The model under review builds one solid part; all positions refer to its coordinate system, in mm. Face numbers are marked on the shaded views. Give positions to 0.01 mm unless a question says otherwise; leave off trailing zeros. Order: outer loops, then holes, each group sorted by start corner. A loop starts at its lowest first (then second) coordinate and runs counter-clockwise, first axis right, second up. Notation, with made-up numbers: M 43.5,78.5 L 62.5,78.5 A25 ccw 62.5,102.5 Z; hole C 19.25,63 d4. An arc over 180 degrees is marked long. One line per question, with ' | ' between items. Start each with the question number.
1. Wall thickness on L1, parallel to Y at x = 0, z = 8.8; L2, parallel to X at y = -21.5, z = 8.5; L3, parallel to X at y = 38.5, z = 6.5: over which ranges is each line inside the solid? List them lowest first.
2. The part is to be moulded in two halves that separate along Y. For the marked faces 1, 2 and 3, say which applies: +Y half, -Y half, draft (parallel to the pull), parting line (faces both ways), or undercut.
3. Insertion check: P1, Ø6, axis at y = 19.5, z = 9, coming from the +X side; P2, Ø4, axis at x = -66.57, y = 21.63, coming from the -Z side; P3, Ø3, axis at x = -19.5, z = 7, coming from the +Y side; P4, Ø6, axis at y = 38, z = 2.5, coming from the -X side. Each pin has a flat end and moves straight along its axis. Give the tip position at first contact, or say it passes through.
4. We need section D-D on z = 3.75. Write out the cut boundary in (x, y), then the cut area to 3 significant figures.
5. We need section B-B on y = 33. Write out the cut boundary in (x, z), then the cut area to 3 significant figures.
6. We need section C-C on x = -53. Write out the cut boundary in (y, z).
7. We need section A-A on x = 0. Write out the cut boundary in (y, z), then the cut area to 3 significant figures.
```python
from build123d import *

# Parameters (mm, degrees)
SKETCH2_R           = 75
BOSS_EXTRUDE1_DEPTH = 10
SKETCH3_R           = 55
CUT_EXTRUDE1_DEPTH  = 10
SKETCH6_R           = 3
CUT_EXTRUDE2_DEPTH  = 3
SKETCH5_R           = 2.5
CUT_EXTRUDE3_DEPTH  = 107.536378763
CIRPATTERN2_COUNT   = 5


with BuildPart() as part:
    # Sketch2 → Boss-Extrude1 (new body)
    with BuildSketch(Plane(origin=(0, 0, 0), x_dir=(0, 1, 0), z_dir=(0, 0, 1))):
        with Locations(Location((0, 0, 0), (0, 0, 270))):
            Circle(SKETCH2_R)
    extrude(amount=BOSS_EXTRUDE1_DEPTH)

    # Sketch3 → Cut-Extrude1 (cut)
    with BuildSketch(Plane.XY.offset(10)):
        Circle(SKETCH3_R)
    extrude(amount=-CUT_EXTRUDE1_DEPTH, mode=Mode.SUBTRACT)

    # Sketch6 → Cut-Extrude2 (cut)
    with BuildSketch(Plane.XY.offset(10)):
        with Locations((0, 70)):
            Circle(SKETCH6_R)
    cut_extrude2 = extrude(amount=-CUT_EXTRUDE2_DEPTH, mode=Mode.SUBTRACT)

    # Sketch5 → Cut-Extrude3 (cut, through all)
    with BuildSketch(Plane.XY.offset(10)):
        with Locations((0, 70)):
            Circle(SKETCH5_R)
    cut_extrude3 = extrude(amount=-CUT_EXTRUDE3_DEPTH, mode=Mode.SUBTRACT)

    # CirPattern2: Cut-Extrude2, Cut-Extrude3 ×5 about axis
    cirpattern2_axis = Axis((0, 0, 0), (0, 0, 1))
    add([cut_extrude2.rotate(cirpattern2_axis, i * 360 / CIRPATTERN2_COUNT) for i in range(1, CIRPATTERN2_COUNT)], mode=Mode.SUBTRACT)
    add([cut_extrude3.rotate(cirpattern2_axis, i * 360 / CIRPATTERN2_COUNT) for i in range(1, CIRPATTERN2_COUNT)], mode=Mode.SUBTRACT)


solid = part.part
```
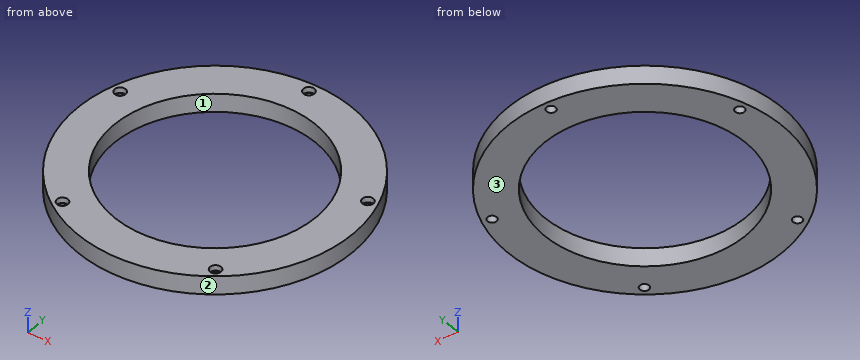
Entries:
1) L1: y = -75 to -55, 55 to 67, 73 to 75 | L2: x = -71.85 to -50.62, 50.62 to 71.85 | L3: x = -64.36 to -39.28, 39.28 to 64.36
2) face 1: undercut | face 2: parting line | face 3: draft
3) P1: stops at x = 73.16 | P2: passes through | P3: stops at y = 72.81 | P4: stops at x = -66.33
4) outline: C 0,0 d150; hole C -66.57,21.63 d5; hole C 0,0 d110; hole C -41.14,-56.63 d5; hole C 0,70 d5; hole C 41.14,-56.63 d5; hole C 66.57,21.63 d5 | area: 8,070 mm^2
5) outline: M -67.35,0 L -44,0 L -44,10 L -67.35,10 Z; M 44,0 L 67.35,0 L 67.35,10 L 44,10 Z | area: 467 mm^2
6) outline: M -53.07,0 L -14.7,0 L -14.7,10 L -53.07,10 Z; M 14.7,0 L 53.07,0 L 53.07,10 L 14.7,10 Z
7) outline: M -75,0 L -55,0 L -55,10 L -75,10 Z; M 55,0 L 67.5,0 L 67.5,7 L 67,7 L 67,10 L 55,10 Z; M 72.5,0 L 75,0 L 75,10 L 73,10 L 73,7 L 72.5,7 Z | area: 347 mm^2
